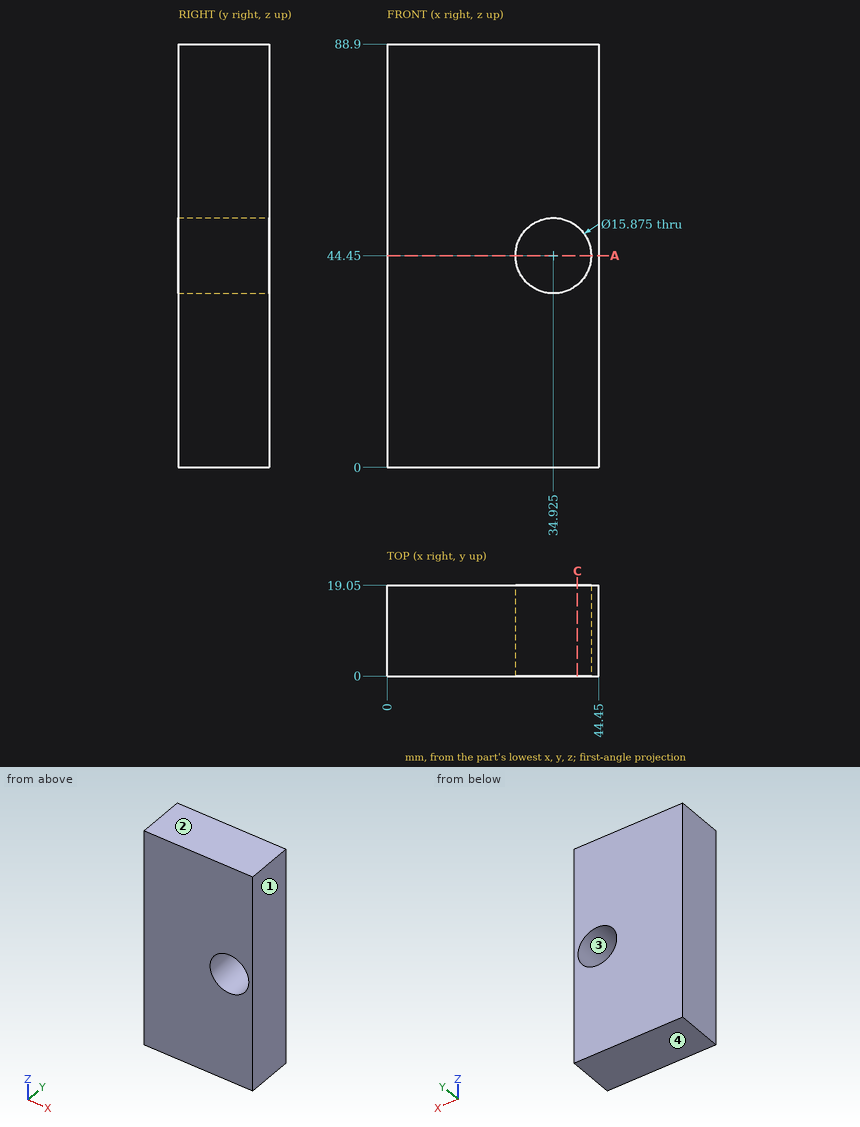
Verification items for this drawing (mm, ordinates from the low corner). Give positions to 0.01 mm unless a question says otherwise; leave off trailing zeros. Loops run counter-clockwise (first coordinate to the right, second up) from the corner with the lowest first, then second, coordinate; pieces in that order, holes last. Notation, with made-up numbers: M 88,-38 L 144,-38 A3 ccw 144,-34 Z; hole C 87.5,47 d7. An arc over 180 degrees is marked long. Write each question's results on one line, items separated by ' | '.
1) Section check A-A, the plane z = 44.45. Record the boundary of the cut face in (x, y), plus the area to 3 significant figures.
Answers follow:
outline: M 0,0 L 26.99,0 L 26.99,19.05 L 0,19.05 Z; M 42.86,0 L 44.45,0 L 44.45,19.05 L 42.86,19.05 Z | area: 544 mm2
2) Section check C-C, the plane x = 40. Record the boundary of the cut face in (y, z), plus the area to 3 significant figures.
Answers follow:
outline: M 0,0 L 19.05,0 L 19.05,38.35 L 0,38.35 Z; M 0,50.55 L 19.05,50.55 L 19.05,88.9 L 0,88.9 Z | area: 1,460 mm2
3) Release check for a two-part mould opening along Z. For the marked faces 1, 2, 3 and 4 record: +Z half, -Z half, draft (parallel to the pull), parting line (faces both ways), or undercut.
Answers follow:
face 1: draft | face 2: +Z half | face 3: undercut | face 4: -Z half
4) Gauge pin test, flat end, axial feed: pin 1 (12.5 mm diameter, centred on x = 34.925, z = 44.45, fed in from -Y). Record the tip position at first contact, or that the pin passes through.
Answers follow:
pin 1: through
5) Thickness scan on line 1 (X direction, y = 15.25, z = 44.45); line 2 (X direction, y = 14.25, z = 43); line 3 (Z direction, x = 29.5, y = 6.75). Record the ranges inside material, lowest first.
Answers follow:
line 1: 0 to 26.99, 42.86 to 44.45 | line 2: 0 to 27.12, 42.73 to 44.45 | line 3: 0 to 38.66, 50.24 to 88.9
